from build123d import *

# Parameters (mm, degrees)
F1_DEPTH  = 9.525
F3_DEPTH  = 6.35
F5_DEPTH  = 6.35
F7_DEPTH  = 6.35
F9_DEPTH  = 6.35
F11_DEPTH = 6.35
F13_DEPTH = 6.35
F15_DEPTH = 6.35
F17_DEPTH = 6.35
F19_DEPTH = 3.175
F20_R     = 5.08


# Not quite as in the source:
# - a feature names something its author has since deleted; it is built from what else it names


with BuildPart() as f1:
    # F0 (on Top) → F1 (new body, symmetric)
    with BuildSketch(Plane.XY):
        Polygon((-32.7905689314, 19.40073682), (-40.8266172422, 5.8184384507), (-36.9048262157, -9.4680410849), (0, 0), align=None)
        Polygon((-24.7545206205, 32.9830351893), (-32.7905689314, 19.40073682), (0, 0), (-9.4680410849, 36.9048262157), align=None)
        Polygon((-9.4680410849, 36.9048262157), (0, 0), (19.40073682, 32.7905689314), (5.8184384507, 40.8266172422), align=None)
        Polygon((19.40073682, 32.7905689314), (0, 0), (36.9048262157, 9.4680410849), (32.9830351893, 24.7545206205), align=None)
        Polygon((36.9048262157, 9.4680410849), (0, 0), (32.7905689314, -19.40073682), (40.8266172422, -5.8184384507), align=None)
        Polygon((32.7905689314, -19.40073682), (0, 0), (9.4680410849, -36.9048262157), (24.7545206205, -32.9830351893), align=None)
        Polygon((9.4680410849, -36.9048262157), (0, 0), (-19.40073682, -32.7905689314), (-5.8184384507, -40.8266172422), align=None)
        Polygon((0, 0), (-36.9048262157, -9.4680410849), (-32.9830351893, -24.7545206205), (-19.40073682, -32.7905689314), align=None)
    extrude(amount=F1_DEPTH, both=True)

    # F2 (on face) → F3 (cut)
    with BuildSketch(Plane(origin=(-36.9048262157, -9.4680410849, 0), x_dir=(0.2485050154, -0.9686306093, 0), z_dir=(-0.9686306093, -0.2485050154, 0))):
        Polygon((-2.794, 0), (-2.794, -2.521839), (-2.794, -5.043678), (2.794, -5.043678), (2.794, -2.521839), (2.794, 0), align=None)
        Polygon((-2.413, 1.556766), (0, 1.556766), (2.413, 1.556766), (2.413, 4.604766), (-2.413, 4.604766), align=None)
    extrude(amount=-F3_DEPTH, mode=Mode.SUBTRACT)

    # F4 (on face) → F5 (cut)
    with BuildSketch(Plane(origin=(-9.4680410849, 36.9048262157, 0), x_dir=(-0.9686306093, -0.2485050154, 0), z_dir=(-0.2485050154, 0.9686306093, 0))):
        Polygon((-2.794, -5.043678), (0, -5.043678), (2.794, -5.043678), (2.794, 0.036322), (0, 0), (-2.794, 0.036322), align=None)
        Polygon((-2.413, 1.593088), (0, 1.593088), (2.413, 1.593088), (2.413, 4.641088), (0, 4.641088), (-2.413, 4.641088), align=None)
    extrude(amount=-F5_DEPTH, mode=Mode.SUBTRACT)

    # F6 (on face) → F7 (cut)
    with BuildSketch(Plane(origin=(-32.7905689314, 19.40073682, 0), x_dir=(-0.5092056908, -0.8606448538, 0), z_dir=(-0.8606448538, 0.5092056908, 0))):
        Polygon((-2.413, 1.593088), (0, 1.593088), (2.413, 1.593088), (2.413, 4.641088), (0, 4.641088), (-2.413, 4.641088), align=None)
        Polygon((-2.794, -5.043678), (0, -5.043678), (2.794, -5.043678), (2.793763897, 0), (-2.793763897, 0), align=None)
    extrude(amount=-F7_DEPTH, mode=Mode.SUBTRACT)

    # F8 (on face) → F9 (cut)
    with BuildSketch(Plane(origin=(19.40073682, 32.7905689314, 0), x_dir=(-0.8606448538, 0.5092056908, 0), z_dir=(0.5092056908, 0.8606448538, 0))):
        Polygon((-2.413, 1.62941), (0, 1.62941), (2.413, 1.62941), (2.413, 4.67741), (-2.413, 4.67741), align=None)
        Polygon((-2.794, -5.043678), (0, -5.043678), (2.794, -5.043678), (2.794, 0.036322), (-2.794, 0.036322), align=None)
    extrude(amount=-F9_DEPTH, mode=Mode.SUBTRACT)

    # F10 (on face) → F11 (cut)
    with BuildSketch(Plane(origin=(36.9048262157, 9.4680410849, 0), x_dir=(-0.2485050154, 0.9686306093, 0), z_dir=(0.9686306093, 0.2485050154, 0))):
        Polygon((-2.794, -4.6912106667), (0, -4.6912106667), (2.794, -4.6912106667), (2.794, 0.3887893333), (-2.794, 0.3887893333), align=None)
        Polygon((-2.413, 1.9818773333), (0, 1.9818773333), (2.413, 1.9818773333), (2.413, 5.0298773333), (-2.413, 5.0298773333), align=None)
    extrude(amount=-F11_DEPTH, mode=Mode.SUBTRACT)

    # F12 (on face) → F13 (cut)
    with BuildSketch(Plane(origin=(32.7905689314, -19.40073682, 0), x_dir=(0.5092056908, 0.8606448538, 0), z_dir=(0.8606448538, -0.5092056908, 0))):
        Polygon((-2.7940002649, -4.4215812), (-2.649e-07, -4.4215812), (2.7939997351, -4.4215812), (2.7939997351, 0.6584188), (-2.649e-07, 0.6220968), (-2.7940002649, 0.6584188), align=None)
        Polygon((-2.4130002649, 2.2151848), (-2.649e-07, 2.2151848), (2.4129997351, 2.2151848), (2.4129997351, 5.2631848), (-2.649e-07, 5.2631848), (-2.4130002649, 5.2631848), align=None)
    extrude(amount=-F13_DEPTH, mode=Mode.SUBTRACT)

    # F14 (on face) → F15 (cut)
    with BuildSketch(Plane(origin=(9.4680410849, -36.9048262157, 0), x_dir=(0.9686306093, 0.2485050154, 0), z_dir=(0.2485050154, -0.9686306093, 0))):
        Polygon((-2.7940002649, -4.4215812), (-2.649e-07, -4.4215812), (2.7939997351, -4.4215812), (2.7939997351, 0.6584188), (-2.649e-07, 0.6220968), (-2.7940002649, 0.6584188), align=None)
        Polygon((-2.4130002649, 2.2151848), (-2.649e-07, 2.2151848), (2.4129997351, 2.2151848), (2.4129997351, 5.2631848), (-2.649e-07, 5.2631848), (-2.4130002649, 5.2631848), align=None)
    extrude(amount=-F15_DEPTH, mode=Mode.SUBTRACT)

    # F16 (on face) → F17 (cut)
    with BuildSketch(Plane(origin=(-19.40073682, -32.7905689314, 0), x_dir=(0.8606448538, -0.5092056908, 0), z_dir=(-0.5092056908, -0.8606448538, 0))):
        Polygon((-2.4130002649, 2.2151848), (-2.649e-07, 2.2151848), (2.4129997351, 2.2151848), (2.4129997351, 5.2631848), (-2.649e-07, 5.2631848), (-2.4130002649, 5.2631848), align=None)
        Polygon((-2.7940002649, -4.4215812), (-2.649e-07, -4.4215812), (2.7939997351, -4.4215812), (2.7939997351, 0.6584188), (-2.649e-07, 0.6220968), (-2.7940002649, 0.6584188), align=None)
    extrude(amount=-F17_DEPTH, mode=Mode.SUBTRACT)

    # F18 (on face) → F19 (join)
    with BuildSketch(Plane.XY.offset(9.525)):
        Polygon((-3.156013695, 12.3016087386), (-15.856013695, 9.0433866005), (-9.543986305, -15.5598308767), (3.156013695, -12.3016087386), (15.856013695, -9.0433866005), (9.543986305, 15.5598308767), align=None)
    extrude(amount=F19_DEPTH)

    # F20
    f20_edges = [f1.edges().sort_by_distance(p)[0] for p in [
        (-5.818438, -40.826617, 0),
        (24.754521, -32.983035, 0),
        (40.826617, -5.818438, 0),
        (32.983035, 24.754521, 0),
        (5.818438, 40.826617, 0),
        (-24.754521, 32.983035, 0),
        (-40.826617, 5.818438, 0),
        (-32.983035, -24.754521, 0),
    ]]
    fillet(f20_edges, radius=F20_R)


solid = f1.part
Source: CAD feature listing. Evaluate the final solid. Frame: model axes, mm. A direction names the side the tool comes from. Round coordinates to 2 decimals unless told otherwise and drop trailing zeros. Order: outer loops, then holes, each group sorted by start corner. A loop starts at its lowest first (then second) coordinate and runs counter-clockwise, first axis right, second up. Notation, with made-up numbers: (16, 63) - (45, 63) arc R24 ccw to (45, 99) - close; hole circle Ø7 at (33.25, 12). An arc over 180 degrees is marked (long way). Use a Markdown table: item, result. Add a question column.
1. Line query: probe 1 along Z at (x, y) = (22.5, -18) (3 decimals); probe 2 along X at (y, z) = (30, 2.5); probe 3 along Y at (x, z) = (-33, -2.5). Output: solid intervals per line, ascending.
2. Section query B-B (y = -2). Return the cut outline in (x, z) (3 decimals), then the cut area to 3 significant figures.
3. Section query C-C (x = 1). Return the cut outline in (y, z) (3 decimals).
4. Mould query, pull axis Y, two halves, no side actions, for faces 1 (the flat face through (17, 1, 9.525)), 2 (the flat face through (-12.744, -3.086, 11.09)), 3 (the flat face through (30, -18, 5.263)). Classes: +Y half, -Y half, draft (parallel to the pull), parting line (faces both ways), or undercut.
5. First-contact query: pin 1 (10 mm diameter, centred on x = 6.5, z = -1, fed in from -Y); pin 2 (4 mm diameter, centred on y = -30.5, z = -2.5, fed in from -X); pin 3 (1 mm diameter, centred on y = 30.5, z = -6.5, fed in from -X). Flat tips, straight axial feed; report the tip coordinate or a pass-through.
6. Section query A-A (z = 7). Return the cut outline in (x, y), then the cut area to 3 significant figures.
7. Set-up query: faces 4 (the flat face through (33.273, 11.027, 3.485)), 5 (the flat face through (-33.2, -11.4, -2.6)), 6 (the flat face through (9, -34, 5.263)). Return all of +Z, -Z, +X, -X, +Y, -Y with unobstructed straight access to the full face (end or side cutting, diameter ignored); none if empty.
8. Section query D-D (x = 24). Return the cut outline in (y, z) (3 decimals).
Derived:
| question | item | result |
|---|---|---|
| 1 | probe 1 | -9.525 to 9.525 |
| 1 | probe 2 | -26.52 to 14.95, 20.55 to 24.12 |
| 1 | probe 3 | -23.97 to -11.35, -5.58 to 16.28 |
| 2 | outline | (-38.821, -9.525) - (39.847, -9.525) - (39.847, 9.525) - (14.049, 9.525) - (14.049, 12.7) - (-13.023, 12.7) - (-13.023, 9.525) - (-38.821, 9.525) - close |
| 2 | area | 1,580 mm2 |
| 3 | outline | (-39.077, -9.525) - (39.59, -9.525) - (39.59, 9.525) - (13.368, 9.525) - (13.368, 12.7) - (-12.855, 12.7) - (-12.855, 9.525) - (-39.077, 9.525) - close |
| 4 | face 1 | draft |
| 4 | face 2 | -Y half |
| 4 | face 3 | undercut |
| 5 | pin 1 | y = -38.95 |
| 5 | pin 2 | x = -26.65 |
| 5 | pin 3 | x = -26.52 |
| 6 | outline | (-40.3, 3.78) - (-33.51, -22.72) arc R5.08 ccw to (-31.17, -25.83) - (-7.63, -39.76) arc R5.08 ccw to (-3.78, -40.3) - (22.72, -33.51) arc R5.08 ccw to (25.83, -31.17) - (39.76, -7.63) arc R5.08 ccw to (40.3, -3.78) - (33.51, 22.72) arc R5.08 ccw to (31.17, 25.83) - (7.63, 39.76) arc R5.08 ccw to (3.78, 40.3) - (-22.72, 33.51) arc R5.08 ccw to (-25.83, 31.17) - (-39.76, 7.63) arc R5.08 ccw to start |
| 6 | area | 4,810 mm2 |
| 7 | face 4 | +X |
| 7 | face 5 | -X |
| 7 | face 6 | none |
| 8 | outline | (-32.981, -9.525) - (30.069, -9.525) - (30.069, 9.525) - (-32.981, 9.525) - close |
